Check sheet for the modelled part. Datum: model origin and axes. Units: mm. Face numbers are marked on the shaded views. A direction names the side the tool comes from. Round coordinates to 2 decimals unless told otherwise and drop trailing zeros. Loops run counter-clockwise (first coordinate to the right, second up) from the corner with the lowest first, then second, coordinate; pieces in that order, holes last. Notation, with made-up numbers: (77.25, 49) - (125.25, 49) arc R21 ccw to (125.25, 61) - close; hole circle Ø10 at (-15.75, 1.25). An arc over 180 degrees is marked (long way). Put each result on its own line as item: value. Start each with the question number.
Item 1: Section check C-C, the plane x = -8. Record the cut outline in (y, z).
Item 2: Section check A-A, the plane z = -4.5. Record the cut outline in (x, y).
Item 3: Tool access check on the marked faces 5, 6 and 7. Record the directions out of +Z, -Z, +X, -X, +Y, -Y that give a thin tool (end or side, any length) a straight path to the whole face; none if there is none.
Item 4: Section check B-B, the plane y = 45.5. Record the cut outline in (x, z), and give its area (3 significant figures).
Item 5: Material ranges on line 1 along Y through (x, z) = (6.5, -4.25); line 2 along X through (y, z) = (-23.5, -7.25); line 3 along Y through (x, z) = (9, 1), recorded low to high.
Item 6: Draft check along X on the marked faces 1, 2, 3 and 4. Enter one of: pulls with the +X half, pulls with the -X half, needs draft (parallel to the pull), parting line crosses it, or undercut.
Item 7: Gauge pin test, flat ends, axial feed: pin 1 Ø5 at (y, z) = (12.5, -4) entering from -X; pin 2 Ø6 at (y, z) = (48, 0.5) entering from +X; pin 3 Ø3 at (x, y) = (7.5, 62.01) entering from -Z; pin 4 Ø2 at (y, z) = (-43.5, 2.5) entering from -X. Record the tip position at first contact, or that the pin passes through.
from build123d import *

# Parameters (mm, degrees)
PAD_DEPTH       = 2
PAD001_DEPTH    = 2
PAD002_DEPTH    = 12
POCKET_DEPTH    = 2
PAD003_DEPTH    = 2
POCKET001_DEPTH = 2
POCKET002_DEPTH = 2
SKETCH004_W     = 23.47
SKETCH004_H     = 24
SKETCH004_W_2   = 24
SKETCH004_H_2   = 23.47
PAD004_DEPTH    = 2
FILLET_R        = 5
FILLET001_R     = 5
FILLET002_R     = 5
SKETCH005_R     = 2
POCKET003_DEPTH = 5


with BuildPart() as part:
    # Sketch → Pad (new body)
    with BuildSketch(Plane.XY):
        with BuildLine():
            Line((-4.211124, 19.211124), (2.610988, 51.047645))
            ThreePointArc((12.389012, 51.047645), (7.5, 55), (2.610988, 51.047645))
            Line((12.389012, 51.047645), (19.211124, 19.211124))
            Line((51.047645, 12.389012), (19.211124, 19.211124))
            ThreePointArc((51.047645, 2.610988), (55, 7.5), (51.047645, 12.389012))
            Line((19.211124, -4.211124), (51.047645, 2.610988))
            Line((12.389012, -36.047645), (19.211124, -4.211124))
            ThreePointArc((2.610988, -36.047645), (7.5, -40), (12.389012, -36.047645))
            Line((-4.211124, -4.211124), (2.610988, -36.047645))
            Line((-4.211124, -4.211124), (-36.047645, 2.610988))
            ThreePointArc((-36.047645, 12.389012), (-40, 7.5), (-36.047645, 2.610988))
            Line((-36.047645, 12.389012), (-4.211124, 19.211124))
        make_face()
        Polygon((15, 0), (50, 7.5), (15, 15), (7.5, 50), (0, 15), (-35, 7.5), (0, 0), (7.5, -35), align=None, mode=Mode.SUBTRACT)
    extrude(amount=PAD_DEPTH)

    # Sketch002 (on Face22 of Pad) → Pad001 (join)
    with BuildSketch(Plane.XY.offset(2)):
        with BuildLine():
            Line((-5.895573, 20.895573), (0.655383, 51.466704))
            ThreePointArc((14.344617, 51.466704), (7.5, 57), (0.655383, 51.466704))
            Line((14.344617, 51.466704), (20.895573, 20.895573))
            Line((51.466704, 14.344617), (20.895573, 20.895573))
            ThreePointArc((51.466704, 0.655383), (57, 7.5), (51.466704, 14.344617))
            Line((20.895573, -5.895573), (51.466704, 0.655383))
            Line((20.895573, -5.895573), (14.344617, -36.466704))
            ThreePointArc((0.655383, -36.466704), (7.5, -42), (14.344617, -36.466704))
            Line((0.655383, -36.466704), (-5.895573, -5.895573))
            Line((-5.895573, -5.895573), (-36.466704, 0.655383))
            ThreePointArc((-36.466704, 14.344617), (-42, 7.5), (-36.466704, 0.655383))
            Line((-5.895573, 20.895573), (-36.466704, 14.344617))
        make_face()
        Polygon((7.5, 50), (15, 15), (50, 7.5), (15, 0), (7.5, -35), (0, 0), (-35, 7.5), (0, 15), align=None, mode=Mode.SUBTRACT)
    extrude(amount=PAD001_DEPTH)

    # Pad001 Face5 → Pad002 (add)
    with BuildSketch(Plane(origin=(7.5, 7.5, 2), x_dir=(0, -1, 0), z_dir=(0, 0, -1))):
        with BuildLine():
            Line((-13.395573, 13.395573), (-43.966704, 6.844617))
            ThreePointArc((-43.966704, 6.844617), (-49.5, 0), (-43.966704, -6.844617))
            Line((-43.966704, -6.844617), (-13.395573, -13.395573))
            Line((-13.395573, -13.395573), (-6.844617, -43.966704))
            ThreePointArc((-6.844617, -43.966704), (0, -49.5), (6.844617, -43.966704))
            Line((6.844617, -43.966704), (13.395573, -13.395573))
            Line((13.395573, -13.395573), (43.966704, -6.844617))
            ThreePointArc((43.966704, -6.844617), (49.5, 0), (43.966704, 6.844617))
            Line((43.966704, 6.844617), (13.395573, 13.395573))
            Line((13.395573, 13.395573), (6.844617, 43.966704))
            ThreePointArc((6.844617, 43.966704), (0, 49.5), (-6.844617, 43.966704))
            Line((-6.844617, 43.966704), (-13.395573, 13.395573))
        make_face()
        with BuildLine():
            Line((-11.711124, 11.711124), (-4.889012, 43.547645))
            ThreePointArc((-4.889012, 43.547645), (0, 47.5), (4.889012, 43.547645))
            Line((4.889012, 43.547645), (11.711124, 11.711124))
            Line((11.711124, 11.711124), (43.547645, 4.889012))
            ThreePointArc((43.547645, 4.889012), (47.5, 0), (43.547645, -4.889012))
            Line((43.547645, -4.889012), (11.711124, -11.711124))
            Line((11.711124, -11.711124), (4.889012, -43.547645))
            ThreePointArc((4.889012, -43.547645), (0, -47.5), (-4.889012, -43.547645))
            Line((-4.889012, -43.547645), (-11.711124, -11.711124))
            Line((-11.711124, -11.711124), (-43.547645, -4.889012))
            ThreePointArc((-43.547645, -4.889012), (-47.5, 0), (-43.547645, 4.889012))
            Line((-43.547645, 4.889012), (-11.711124, 11.711124))
        make_face(mode=Mode.SUBTRACT)
    extrude(amount=PAD002_DEPTH)

    # Pad002 Face23 → Pocket (cut)
    with BuildSketch(Plane(origin=(7.5, 7.5, 4), x_dir=(0, 1, 0), z_dir=(0, 0, 1))):
        with BuildLine():
            Line((43.966704, 6.844617), (13.395573, 13.395573))
            Line((13.395573, 13.395573), (6.844617, 43.966704))
            ThreePointArc((6.844617, 43.966704), (0, 49.5), (-6.844617, 43.966704))
            Line((-6.844617, 43.966704), (-13.395573, 13.395573))
            Line((-13.395573, 13.395573), (-43.966704, 6.844617))
            ThreePointArc((-43.966704, 6.844617), (-49.5, 0), (-43.966704, -6.844617))
            Line((-43.966704, -6.844617), (-13.395573, -13.395573))
            Line((-13.395573, -13.395573), (-6.844617, -43.966704))
            ThreePointArc((-6.844617, -43.966704), (0, -49.5), (6.844617, -43.966704))
            Line((6.844617, -43.966704), (13.395573, -13.395573))
            Line((13.395573, -13.395573), (43.966704, -6.844617))
            ThreePointArc((43.966704, -6.844617), (49.5, 0), (43.966704, 6.844617))
        make_face()
        Polygon((42.5, 0), (7.5, -7.5), (0, -42.5), (-7.5, -7.5), (-42.5, 0), (-7.5, 7.5), (0, 42.5), (7.5, 7.5), align=None, mode=Mode.SUBTRACT)
    extrude(amount=-POCKET_DEPTH, mode=Mode.SUBTRACT)

    # Sketch003 (on Face23 of Pocket) → Pad003 (join)
    with BuildSketch(Plane.XY.offset(2)):
        with BuildLine():
            Line((-10.106697, 25.106697), (-4.233629, 52.514349))
            ThreePointArc((19.233629, 52.514349), (7.5, 62), (-4.233629, 52.514349))
            Line((19.233629, 52.514349), (25.106697, 25.106697))
            Line((25.106697, 25.106697), (52.514349, 19.233629))
            ThreePointArc((52.514349, -4.233629), (62, 7.5), (52.514349, 19.233629))
            Line((52.514349, -4.233629), (25.106697, -10.106697))
            Line((25.106697, -10.106697), (19.233629, -37.514349))
            ThreePointArc((-4.233629, -37.514349), (7.5, -47), (19.233629, -37.514349))
            Line((-4.233629, -37.514349), (-10.106697, -10.106697))
            Line((-10.106697, -10.106697), (-37.514349, -4.233629))
            ThreePointArc((-37.514349, 19.233629), (-47, 7.5), (-37.514349, -4.233629))
            Line((-37.514349, 19.233629), (-10.106697, 25.106697))
        make_face()
        Polygon((7.5, 50), (15, 15), (50, 7.5), (15, 0), (7.5, -35), (0, 0), (-35, 7.5), (0, 15), align=None, mode=Mode.SUBTRACT)
    extrude(amount=PAD003_DEPTH)

    # Pad003 Face1 → Pocket001 (cut)
    with BuildSketch(Plane(origin=(7.5, 7.5, 0), x_dir=(0, -1, 0), z_dir=(0, 0, -1))):
        with BuildLine():
            Line((-11.711124, 11.711124), (-43.547645, 4.889012))
            ThreePointArc((-43.547645, 4.889012), (-47.5, 0), (-43.547645, -4.889012))
            Line((-43.547645, -4.889012), (-11.711124, -11.711124))
            Line((-11.711124, -11.711124), (-4.889012, -43.547645))
            ThreePointArc((-4.889012, -43.547645), (0, -47.5), (4.889012, -43.547645))
            Line((4.889012, -43.547645), (11.711124, -11.711124))
            Line((11.711124, -11.711124), (43.547645, -4.889012))
            ThreePointArc((43.547645, -4.889012), (47.5, 0), (43.547645, 4.889012))
            Line((43.547645, 4.889012), (11.711124, 11.711124))
            Line((11.711124, 11.711124), (4.889012, 43.547645))
            ThreePointArc((4.889012, 43.547645), (0, 47.5), (-4.889012, 43.547645))
            Line((-4.889012, 43.547645), (-11.711124, 11.711124))
        make_face()
        Polygon((7.5, 7.5), (42.5, 0), (7.5, -7.5), (0, -42.5), (-7.5, -7.5), (-42.5, 0), (-7.5, 7.5), (0, 42.5), align=None, mode=Mode.SUBTRACT)
    extrude(amount=-POCKET001_DEPTH, mode=Mode.SUBTRACT)

    # Pocket001 Face1 → Pocket002 (cut)
    with BuildSketch(Plane(origin=(7.5, 7.5, -10), x_dir=(0, -1, 0), z_dir=(0, 0, -1))):
        with BuildLine():
            Line((-13.395573, 13.395573), (-43.966704, 6.844617))
            ThreePointArc((-43.966704, 6.844617), (-49.5, 0), (-43.966704, -6.844617))
            Line((-43.966704, -6.844617), (-13.395573, -13.395573))
            Line((-13.395573, -13.395573), (-6.844617, -43.966704))
            ThreePointArc((-6.844617, -43.966704), (0, -49.5), (6.844617, -43.966704))
            Line((6.844617, -43.966704), (13.395573, -13.395573))
            Line((13.395573, -13.395573), (43.966704, -6.844617))
            ThreePointArc((43.966704, -6.844617), (49.5, 0), (43.966704, 6.844617))
            Line((43.966704, 6.844617), (13.395573, 13.395573))
            Line((13.395573, 13.395573), (6.844617, 43.966704))
            ThreePointArc((6.844617, 43.966704), (0, 49.5), (-6.844617, 43.966704))
            Line((-6.844617, 43.966704), (-13.395573, 13.395573))
        make_face()
        with BuildLine():
            Line((-11.711124, 11.711124), (-4.889012, 43.547645))
            ThreePointArc((-4.889012, 43.547645), (0, 47.5), (4.889012, 43.547645))
            Line((4.889012, 43.547645), (11.711124, 11.711124))
            Line((11.711124, 11.711124), (43.547645, 4.889012))
            ThreePointArc((43.547645, 4.889012), (47.5, 0), (43.547645, -4.889012))
            Line((43.547645, -4.889012), (11.711124, -11.711124))
            Line((11.711124, -11.711124), (4.889012, -43.547645))
            ThreePointArc((4.889012, -43.547645), (0, -47.5), (-4.889012, -43.547645))
            Line((-4.889012, -43.547645), (-11.711124, -11.711124))
            Line((-11.711124, -11.711124), (-43.547645, -4.889012))
            ThreePointArc((-43.547645, -4.889012), (-47.5, 0), (-43.547645, 4.889012))
            Line((-43.547645, 4.889012), (-11.711124, 11.711124))
        make_face(mode=Mode.SUBTRACT)
    extrude(amount=-POCKET002_DEPTH, mode=Mode.SUBTRACT)

    # Sketch004 (on Face5 of Pocket002) → Pad004 (join)
    with BuildSketch(Plane(origin=(0, 0, 2), x_dir=(1, 0, 0), z_dir=(0, 0, -1))):
        with Locations((7.501371, -64.514349)):
            Rectangle(SKETCH004_W, SKETCH004_H)
        with Locations((64.514349, -7.501371)):
            Rectangle(SKETCH004_W_2, SKETCH004_H_2)
        with Locations((7.501371, 49.514349)):
            Rectangle(SKETCH004_W, SKETCH004_H)
        with Locations((-49.514349, -7.501371)):
            Rectangle(SKETCH004_W_2, SKETCH004_H_2)
    extrude(amount=-PAD004_DEPTH)

    # Fillet
    fillet_edges = [part.edges().sort_by_distance(p)[0] for p in [
        (-61.514349, 19.236371, 3),
        (-61.514349, -4.233629, 3),
    ]]
    fillet(fillet_edges, radius=FILLET_R)

    # Fillet001
    fillet001_edges = [part.edges().sort_by_distance(p)[0] for p in [
        (-4.233629, -61.514349, 3),
        (19.236371, -61.514349, 3),
        (76.514349, -4.233629, 3),
        (76.514349, 19.236371, 3),
    ]]
    fillet(fillet001_edges, radius=FILLET001_R)

    # Fillet002
    fillet002_edges = [part.edges().sort_by_distance(p)[0] for p in [
        (-4.233629, 76.514349, 3),
        (19.236371, 76.514349, 3),
    ]]
    fillet(fillet002_edges, radius=FILLET002_R)

    # Sketch005 (on Face46 of Fillet002) → Pocket003 (cut)
    with BuildSketch(Plane.XY.offset(4)):
        with Locations((7.501371, 62.014349)):
            Circle(SKETCH005_R)
        with Locations((7.501371, -47.014349)):
            Circle(SKETCH005_R)
        with Locations((62.014349, 7.501371)):
            Circle(SKETCH005_R)
        with Locations((-47.014349, 7.501371)):
            Circle(SKETCH005_R)
    extrude(amount=-POCKET003_DEPTH, mode=Mode.SUBTRACT)


solid = part.part
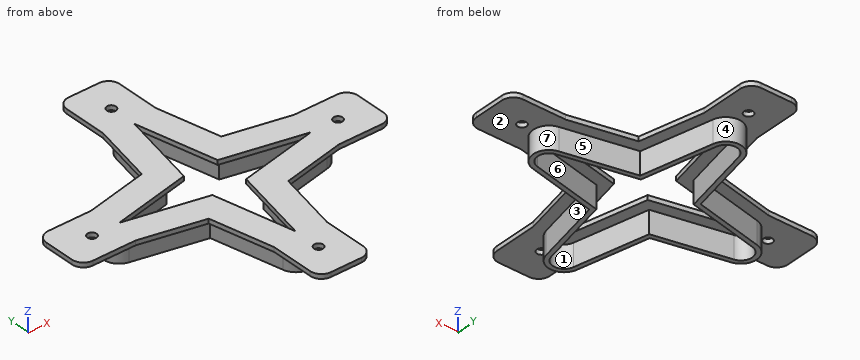
Check result:
1. outline: (-19.94, 2) - (-5.44, 2) - (-5.44, -8) - (-3.4, -8) - (-3.4, 2) - (1.71, 2) - (1.71, 4) - (-19.94, 4) - close; (13.29, 2) - (18.4, 2) - (18.4, -8) - (20.44, -8) - (20.44, 2) - (34.94, 2) - (34.94, 4) - (13.29, 4) - close
2. outline: (-36.47, 0.66) - (-5.9, -5.9) - (0.66, -36.47) arc R7 ccw to (14.34, -36.47) - (20.9, -5.9) - (51.47, 0.66) arc R7 ccw to (51.47, 14.34) - (20.9, 20.9) - (14.34, 51.47) arc R7 ccw to (0.66, 51.47) - (-5.9, 20.9) - (-36.47, 14.34) arc R7 ccw to start; hole (-36.05, 2.61) - (-4.21, -4.21) - (2.61, -36.05) arc R5 ccw to (12.39, -36.05) - (19.21, -4.21) - (51.05, 2.61) arc R5 ccw to (51.05, 12.39) - (19.21, 19.21) - (12.39, 51.05) arc R5 ccw to (2.61, 51.05) - (-4.21, 19.21) - (-36.05, 12.39) arc R5 ccw to start
3. face 5: -Z, +X, +Y
3. face 6: -Z
3. face 7: -Z, +X
4. outline: (-5.74, 2) - (-0.62, 2) - (-0.62, -8) - (1.42, -8) - (1.42, 2) - (6.54, 2) - (6.54, 4) - (-5.74, 4) - close; (8.46, 2) - (13.58, 2) - (13.58, -8) - (15.62, -8) - (15.62, 2) - (20.74, 2) - (20.74, 4) - (8.46, 4) - close
4. area: 90.0 mm²
5. line 1: -41.93 to -39.9, 54.9 to 56.93
5. line 2: -2.12 to -0.08, 15.08 to 17.12
5. line 3: -41.84 to -39.77, 54.77 to 56.84
6. face 1: undercut
6. face 2: needs draft
6. face 3: pulls with the +X half
6. face 4: parting line crosses it
7. pin 1: x = -41.54
7. pin 2: x = 20.76
7. pin 3: through
7. pin 4: x = -4.23
